Source: CAD feature listing. Evaluate the final solid. Frame: model axes, mm. A direction names the side the tool comes from. Round coordinates to 2 decimals unless told otherwise and drop trailing zeros. Loops run counter-clockwise (first coordinate to the right, second up) from the corner with the lowest first, then second, coordinate; pieces in that order, holes last. Notation, with made-up numbers: M 80.25,17.25 L 129.25,17.25 A19 cw 129.25,39.25 Z; hole C -10,-35 d8. An arc over 180 degrees is marked long. Answer as a JSON object with one key per item and string values.
from build123d import *

# Parameters (mm, degrees)
BOSS_EXTRUDE2_DEPTH = 20
FILLET1_RADIUS      = 10
FILLET1_LENGTH      = 5
FILLET2_RADIUS      = 10
FILLET2_LENGTH      = 5
SKETCH5_R           = 1
SKETCH5_R_2         = 5.5
CUT_EXTRUDE5_DEPTH  = 69.007352544
CUT_EXTRUDE7_DEPTH  = 25
FILLET5_R           = 10
BOSS_EXTRUDE5_DEPTH = 60
SKETCH13_R          = 2.1
CUT_EXTRUDE8_DEPTH  = 60


with BuildPart() as part:
    # Sketch1 → Boss-Extrude2 (new body)
    with BuildSketch(Plane.XY):
        Polygon((-25, 30), (25, 30), (25, -30), (-25, -30), (-25, -25), (-20, -25), (20, -25), (20, 25), (-20, 25), (-25, 25), align=None)
    extrude(amount=BOSS_EXTRUDE2_DEPTH)

    # Fillet1: full round fillet: the end face becomes a half cylinder, R = half its width
    fillet1_face = Plane((-25, 27.5, 10), x_dir=(0, -1, 0), z_dir=(-1, 0, 0))  # on the end face: x along it, z out of the body
    fillet1_slab = fillet1_face.offset(-FILLET1_RADIUS / 2) * Box(FILLET1_LENGTH, 2 * FILLET1_RADIUS, FILLET1_RADIUS, mode=Mode.PRIVATE)  # the body's end, R deep
    fillet1_round = Plane((-15, 27.5, 10), x_dir=(-1, 0, 0), z_dir=(0, -1, 0)) * Cylinder(FILLET1_RADIUS, FILLET1_LENGTH, mode=Mode.PRIVATE)  # its axis R under the face
    add(fillet1_slab - fillet1_round, mode=Mode.SUBTRACT)

    # Fillet2: full round fillet: the end face becomes a half cylinder, R = half its width
    fillet2_face = Plane((-25, -27.5, 10), x_dir=(0, -1, 0), z_dir=(-1, 0, 0))  # on the end face: x along it, z out of the body
    fillet2_slab = fillet2_face.offset(-FILLET2_RADIUS / 2) * Box(FILLET2_LENGTH, 2 * FILLET2_RADIUS, FILLET2_RADIUS, mode=Mode.PRIVATE)  # the body's end, R deep
    fillet2_round = Plane((-15, -27.5, 10), x_dir=(-1, 0, 0), z_dir=(0, -1, 0)) * Cylinder(FILLET2_RADIUS, FILLET2_LENGTH, mode=Mode.PRIVATE)  # its axis R under the face
    add(fillet2_slab - fillet2_round, mode=Mode.SUBTRACT)

    # Sketch5 → Cut-Extrude5 (cut, through all)
    with BuildSketch(Plane(origin=(0, 30, 0), x_dir=(1, 0, 0), z_dir=(0, 1, 0))):
        with Locations(Location((-15, -3, 0), (0, 0, 180))):
            Circle(SKETCH5_R)
        with Locations(Location((-22, -10, 0), (0, 0, 180))):
            Circle(SKETCH5_R)
        with Locations(Location((-15, -17, 0), (0, 0, 180))):
            Circle(SKETCH5_R)
        with Locations(Location((-8, -10, 0), (0, 0, 180))):
            Circle(SKETCH5_R)
        with Locations(Location((-15, -10, 0), (0, 0, 180))):
            Circle(SKETCH5_R_2)
    extrude(amount=-CUT_EXTRUDE5_DEPTH, mode=Mode.SUBTRACT)

    # Sketch10 → Cut-Extrude7 (cut)
    with BuildSketch(Plane(origin=(25, 0, 0), x_dir=(0, 0, -1), z_dir=(1, 0, 0))):
        Polygon((-15, 28.180148829), (-15, -28.180148829), (-15, -30), (-20, -30), (-20, 30), (-15, 30), align=None)
        Polygon((-5, 28.180148829), (-5, -28.180148829), (-5, -30), (0, -30), (0, 30), (-5, 30), align=None)
    extrude(amount=-CUT_EXTRUDE7_DEPTH, mode=Mode.SUBTRACT)

    # Fillet5
    # the kernel refuses this fillet: 10 mm, written as the material it adds along each edge
    with BuildSketch(Plane(origin=(0, 25, 15), x_dir=(1, 0, 0), z_dir=(0, 1, 0)), Plane(origin=(0, -30, 15), x_dir=(1, 0, 0), z_dir=(0, 1, 0)), Plane(origin=(0, -25, 5), x_dir=(1, 0, 0), z_dir=(0, -1, 0))) as fillet5_piece_1:
        with BuildLine():
            CenterArc((8.660254038, -10), FILLET5_R, 90, 60)
            Line((0, -5), (-0.173205081, -4.9))
            ThreePointArc((-0.173205081, -4.9), (-0.2, -2.5), (-0.2, 0))
            Line((-0.2, 0), (0, 0.2))
            Line((0, 0.2), (8.660254038, 0.2))
            Line((8.660254038, 0.2), (8.660254038, 0))
        make_face()
    extrude(amount=5)
    with BuildSketch(Plane(origin=(0, 30, 5), x_dir=(0, 0, -1), z_dir=(0, -1, 0))) as fillet5_piece_2:
        with BuildLine():
            CenterArc((10, 8.660254038), FILLET5_R, 180, 60)
            Line((0, 8.660254038), (-0.2, 8.660254038))
            Line((-0.2, 8.660254038), (-0.2, 0))
            Line((-0.2, 0), (0, -0.2))
            ThreePointArc((0, -0.2), (2.5, -0.2), (4.9, -0.173205081))
            Line((4.9, -0.173205081), (5, 0))
        make_face()
    extrude(amount=5)

    # Sketch12 → Boss-Extrude5 (add)
    with BuildSketch(Plane.XZ.offset(30)):
        with BuildLine():
            Line((56.226298398, -3.359735054), (61.222506141, 5.302707337))
            ThreePointArc((61.222506141, 5.302707337), (43.74904955, 12.533728595), (25, 15))
            Line((25, 15), (25, 5))
            ThreePointArc((25, 5), (41.16297375, 2.873903962), (56.226298398, -3.359735054))
        make_face()
    extrude(amount=-BOSS_EXTRUDE5_DEPTH)

    # Sketch13 → Cut-Extrude8 (cut)
    with BuildSketch(Plane(origin=(2.920998947, 0, 10.910870277), x_dir=(-0.9659824633840055, 0, 0.2586075800021504), z_dir=(-0.2586075800021504, 0, -0.9659824633840055))):
        with Locations((-39.019497435, 15)):
            Circle(SKETCH13_R)
        with Locations((-39.019497435, 0)):
            Circle(SKETCH13_R)
        with Locations((-39.019497435, -15)):
            Circle(SKETCH13_R)
    extrude(amount=-CUT_EXTRUDE8_DEPTH, mode=Mode.SUBTRACT)


solid = part.part
Item 1: Access query for faces 4 (the flat face through (-7, 28, 0)), 5 (the flat face through (18, 30, 8)), 6 (the flat face through (20, 0, 10)), 7 (the cylindrical face through (37.404, -0.42, 3.757)), 8 (the cylindrical face through (-25, 27, 10)). Directions: +Z, -Z, +X, -X, +Y, -Y. A direction counts if a zero-diameter tool reaches every point of the face in a straight line with its end or side. Return the directions, or none.
Answer sheet:
{"face 4": "-Z, -X, +Y, -Y", "face 5": "+Z, -Z, +X, -X, +Y", "face 6": "+Z, -Z, -X", "face 7": "-Z, +Y, -Y", "face 8": "-X, +Y, -Y"}
Item 2: Pull-direction query (Z, two-part tool) for faces 1 (the cylindrical face through (-16, 28, 3)), 2 (the flat face through (-2, -25, 10)), 3 (the cylindrical face through (3.724, 27.535, 3.697)); classes: pulls with the +Z half, pulls with the -Z half, needs draft (parallel to the pull), parting line crosses it, or undercut.
Answer sheet:
{"face 1": "undercut", "face 2": "needs draft", "face 3": "pulls with the -Z half"}
Item 3: Line query: probe 1 along Z at (x, y) = (-15, 27); probe 2 along Z at (x, y) = (-8, -28.3); probe 3 along Y at (x, z) = (-21, 14.75). Output: solid intervals per line, ascending. Write a range as from..to.
Answer sheet:
{"probe 1": "z = 0..2, 4..4.5, 15.5..16, 18..20", "probe 2": "z = 0..9, 11..20", "probe 3": "y = -30..-25, 25..30"}
Item 4: Contact query for flat-ended pins moving along their axis: pin 1 Ø5 at (x, y) = (19.5, 13.5) entering from -Z; pin 2 Ø2.5 at (x, y) = (-7, -27) entering from -Z; pin 3 Ø3 at (y, z) = (5, 10) entering from -X. Output: stop coordinate, or through.
Answer sheet:
{"pin 1": "stops at z = 5", "pin 2": "stops at z = 0", "pin 3": "stops at x = 20"}
Item 5: Section B-B on z = 17. Return the cut outline in (x, y).
Answer sheet:
{"outline": "M -22.14,-30 L -16,-30 L -16,-25 L -22.14,-25 Z; M -22.14,25 L -16,25 L -16,30 L -22.14,30 Z; M -14,-30 L 2.66,-30 L 2.66,-25 L -14,-25 Z; M -14,25 L 2.66,25 L 2.66,30 L -14,30 Z"}
Item 6: Section D-D on y = -20.5. Return the cut outline in (x, z), then the cut area to 3 significant figures.
Answer sheet:
{"outline": "M 20,5 L 25,5 A62.5 cw 56.23,-3.36 L 61.22,5.3 A72.5 ccw 25,15 L 20,15 Z", "area": "403 mm²"}
Item 7: Section C-C on x = -8. Return the cut outline in (y, z).
Answer sheet:
{"outline": "M -30,0 L -25,0 L -25,9 L -30,9 Z; M -30,11 L -25,11 L -25,20 L -30,20 Z; M 25,0 L 30,0 L 30,9 L 25,9 Z; M 25,11 L 30,11 L 30,20 L 25,20 Z"}
Item 8: Section A-A on x = 13. Return the cut outline in (y, z), then the cut area to 3 significant figures.
Answer sheet:
{"outline": "M -30,5 L -25,5 L -25,15 L -30,15 Z; M 25,5 L 30,5 L 30,15 L 25,15 Z", "area": "100 mm²"}
